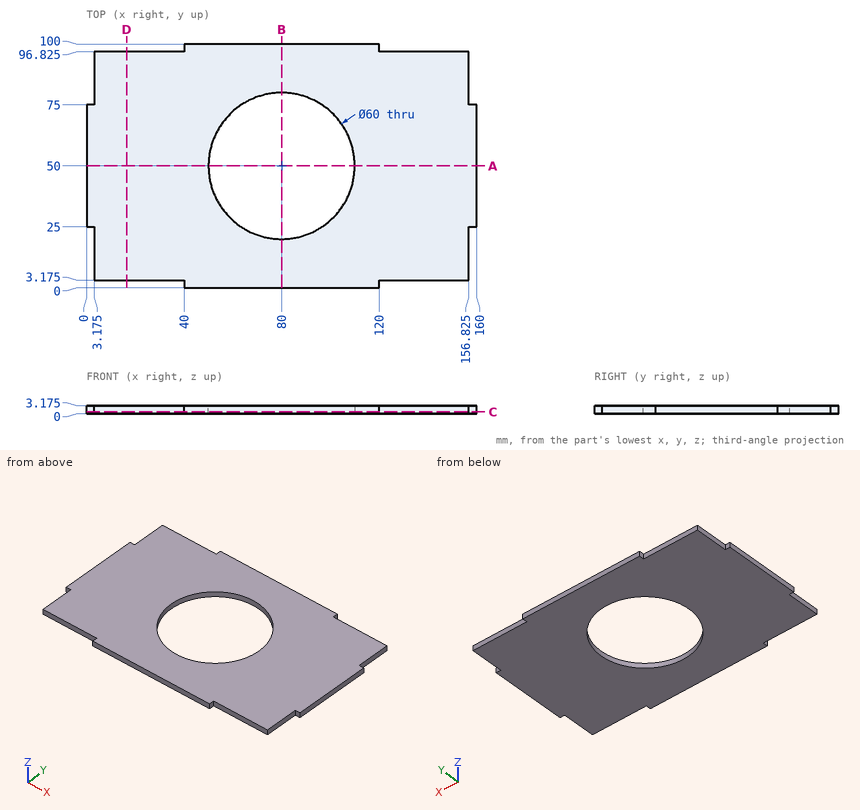
For this review, use the dimensioned drawing (mm, ordinates from the lowest corner) and the shaded views. Give positions to 0.01 mm unless a question says otherwise; leave off trailing zeros. Order: outer loops, then holes, each group sorted by start corner. A loop starts at its lowest first (then second) coordinate and runs counter-clockwise, first axis right, second up. Notation, with made-up numbers: (-7.75, -28) - (-0.75, -28) arc R25 cw to (-0.75, -10) - close; hole circle Ø9 at (34.5, -35). An arc over 180 degrees is marked (long way). Use CSV: the item, a comma, the result in double quotes. Start each with the question number.
Q1. Take a section at D-D (x = 16.5). State the section outline as (y, z) points (3 decimals), and give its area (3 significant figures).
Q2. Take a section at A-A (y = 50). State the section outline as (x, z) points (3 decimals).
Q3. For P1, Ø1, axis at x = 2.5, z = 1, coming from the +Y side; P2, Ø1.6, axis at x = 2, z = 1.5, coming from the -Y side; P3, Ø1.6, axis at y = 87, z = 2.5, coming from the -X side (3 decimals), all flat-tipped, find the tip position at first contact; note any pin that passes through.
Q4. Take a section at C-C (z = 0.7). State the section outline as (x, y) points (3 decimals), and give its area (3 significant figures).
Q5. Take a section at B-B (x = 80). State the section outline as (y, z) points (3 decimals), and give its area (3 significant figures).
Q6. For line 1 (Y direction, x = 80, z = 1.3); line 2 (X direction, y = 83, z = 2.4) (3 decimals); line 3 (X direction, y = 58, z = 0.2), list the stretches that pass through material, from the lowest coordinate up.
Calculated:
1,outline,"(3.175, 0) - (96.825, 0) - (96.825, 3.175) - (3.175, 3.175) - close"
1,area,"297 mm²"
2,outline,"(0, 0) - (50, 0) - (50, 3.175) - (0, 3.175) - close; (110, 0) - (160, 0) - (160, 3.175) - (110, 3.175) - close"
3,P1,"stops at y = 75"
3,P2,"stops at y = 25"
3,P3,"stops at x = 3.175"
4,outline,"(0, 25) - (3.175, 25) - (3.175, 3.175) - (40, 3.175) - (40, 0) - (120, 0) - (120, 3.175) - (156.825, 3.175) - (156.825, 25) - (160, 25) - (160, 75) - (156.825, 75) - (156.825, 96.825) - (120, 96.825) - (120, 100) - (40, 100) - (40, 96.825) - (3.175, 96.825) - (3.175, 75) - (0, 75) - close; hole circle Ø60 at (80, 50)"
4,area,"12,400 mm²"
5,outline,"(0, 0) - (20, 0) - (20, 3.175) - (0, 3.175) - close; (80, 0) - (100, 0) - (100, 3.175) - (80, 3.175) - close"
5,area,"127 mm²"
6,line 1,"y = 0 to 20, 80 to 100"
6,line 2,"x = 3.175 to 156.825"
6,line 3,"x = 0 to 51.09, 108.91 to 160"
